The model under review builds one solid part; all positions refer to its coordinate system, in mm. A direction names the side the tool comes from. Give positions to 0.01 mm unless a question says otherwise; leave off trailing zeros. Loops run counter-clockwise (first coordinate to the right, second up) from the corner with the lowest first, then second, coordinate; pieces in that order, holes last. Notation, with made-up numbers: (36.25, -0.75) - (40.25, -0.75) arc R14 cw to (40.25, 8.25) - close; hole circle Ø1 at (-36.75, -38). An arc over 180 degrees is marked (long way). Return JSON: item names as keys, results as strings. Group by question number.
Autodesk Inventor part; units mm, degrees
ref_plane "YZ Plane" through (0, 0, 0) normal (1, 0, 0) x (0, 1, 0)
ref_plane "XZ Plane" through (0, 0, 0) normal (0, 1, 0) x (-1, 0, 0)
ref_plane "XY Plane" through (0, 0, 0) normal (0, 0, 1) x (1, 0, 0)
sketch "Sketch1" plane through (0, 0, 0) normal (0, 0, 1) x (1, 0, 0)
  circle A0 centre (0, 0) radius 10
  arc A1 (13.1244, -10) -> (-13.1244, -10) centre (0, 0) ccw
  line L0 (13.1244, -10) -> (25, -10)
  line L1 (25, -10) -> (0, -10)
  line L2 (-13.1244, -10) -> (-25, -10)
  line L3 (0, 0) -> (0, -17.5)
  line L4 (0, -17.5) -> (-25, -17.5)
  line L5 (-25, -17.5) -> (-25, -10)
  line L6 (25, -10) -> (25, -17.5)
  line L7 (25, -17.5) -> (0, -17.5)
  line L8 (0, 0) -> (-12.5, 0)
  circle A2 centre (-12.5, 0) radius 1.25
  line L9 (0, 0) -> (0, 12.5)
  circle A3 centre (0, 12.5) radius 1.25
  circle A4 centre (12.5, 0) radius 1.25
  circle A5 centre (0, -12.5) radius 1.25
  circle A6 centre (12.5, 0) radius 3.25
  circle A7 centre (-12.5, 0) radius 3.25
  line L10 (0, 0) -> (2.11, 2.11)
  line L11 (0, 0) -> (2.984, 0) construction
  circle A8 centre (0, 12.5) radius 3.25
  circle A9 centre (0, -12.5) radius 3.25
  dimension "d0" = 20
  dimension "d1" = 33
  dimension "d2" = 25
  dimension "d3" = 25
  dimension "d4" = 17.5
  dimension "d5" = 25
  dimension "d6" = 12.5
  dimension "d7" = 2.5
  dimension "d8" = 12.5
  dimension "d9" = 2.5
  dimension "d15" = 6.5
  dimension "d16" = 45
  dimension "d17" = 6.5
  dimension "d18" = 6.5
extrude "Extrusion1" add sketch "Sketch1" along normal blind 6 contours A0 A6 | A0 A8 A7 A9 L3 L4 L5 L2 A1 L1 A6 | A0 A8 | A9 L1 A0 | L3 A5 A9 A0 | L1 A9 L3 A5 | L1 L0 L6 L7 L3 A9 | A5 L3 | L3 A5 | A0 A7 picked at (10.6028, 1.4923)
fillet "Fillet1" radius 5 2 edges at (13.1244, -10, 3) (-13.1244, -10, 3)
sketch "Sketch2" plane through (0, 0, 0) normal (0, 0, -1) x (-1, 0, 0)
  circle A0 centre (0, 12.5) radius 1.25
  line L0 (0, 0) -> (-3.0567, 0)
  circle A1 centre (0, -12.5) radius 1.25
extrude "Extrusion2" cut sketch "Sketch2" against normal blind 10 contours A1
sketch "Sketch3" plane through (0, 0, 0) normal (0, 0, -1) x (-1, 0, 0)
  circle A0 centre (-12.5, 0) radius 1.25
  circle A1 centre (0, -12.5) radius 1.25
  circle A2 centre (0, 0) radius 10
  circle A3 centre (-12.5, 0) radius 1.25
  circle A4 centre (0, 12.5) radius 1.25
  circle A5 centre (12.5, 0) radius 1.25
  line L0 (25, -17.5) -> (-25, -17.5)
  line L1 (25, -10) -> (25, -17.5)
  line L2 (20.9105, -10) -> (25, -10)
  arc A6 (16.0476, -3.8372) -> (20.9105, -10) centre (20.9105, -5) ccw
  arc A7 (16.0476, -3.8372) -> (-16.0476, -3.8372) centre (0, 0) ccw
  arc A8 (-20.9105, -10) -> (-16.0476, -3.8372) centre (-20.9105, -5) ccw
  line L3 (-25, -10) -> (-20.9105, -10)
  line L4 (-25, -17.5) -> (-25, -10)
  circle A9 centre (-12.5, 0) radius 3.25
  circle A10 centre (0, 12.5) radius 3.25
  circle A11 centre (12.5, 0) radius 1.25
  circle A12 centre (12.5, 0) radius 3.25
  circle A13 centre (0, -12.5) radius 3.25
  dimension "d19" = 6.5
  dimension "d20" = 6.5
  dimension "d21" = 6.5
  dimension "d22" = 6.5
extrude "Extrusion3" cut sketch "Sketch3" against normal blind 3 contours A2 A12 | A2 A12 | A10 A2 | A2 A10 | A13 A2 | A2 A13 | A9 A2 | A2 A9
sketch "Sketch4" plane through (0, 0, 0) normal (0, 0, -1) x (-1, 0, 0)
  arc A0 (16.0476, -3.8372) -> (-16.0476, -3.8372) centre (0, 0) ccw
  line L0 (-25, -10) -> (-20.9105, -10)
  line L1 (-16.0476, 3.8372) -> (-20.9105, -10)
  line L2 (15.5959, 5.3868) -> (20.9105, -10)
  arc A1 (16.0476, -3.8372) -> (20.9105, -10) centre (20.9105, -5) ccw
  arc A2 (-20.9105, -10) -> (-16.0476, -3.8372) centre (-20.9105, -5) ccw
extrude "Extrusion4" add sketch "Sketch4" against normal up to surface (6 mm away)
sketch "Sketch5" plane through (-25, -17.5, 0) normal (0, -1, 0) x (1, 0, 0)
  line L0 (0, 6) -> (50, 6)
  line L1 (0, 0) -> (50, 0)
  circle A0 centre (40.75, 3) radius 1.25
  circle A1 centre (9.25, 3) radius 1.25
  point P0 (25, 0)
  dimension "d27" = 2.5
extrude "Extrusion5" cut sketch "Sketch5" against normal blind 14
sketch "Sketch6" plane through (-25, -17.5, 0) normal (0, -1, 0) x (1, 0, 0)
  circle A0 centre (9.25, 3) radius 1.25
  circle A1 centre (40.75, 3) radius 1.25
  point P0 (25, 0)
  dimension "d30" = 31.5
sketch "Sketch8" plane through (-25, -10, 6) normal (0, 1, 0) x (1, 0, 0)
  line L0 (9.4041, 6) -> (41.0476, 6)
  line L1 (4.0895, 6) -> (4.0895, 0)
  line L2 (9.4041, 6) -> (4.0895, 6)
  line L3 (4.0895, 6) -> (4.0895, 0)
  line L4 (4.0895, 0) -> (9.4041, 0)
  line L5 (9.4041, 0) -> (9.4041, 6)
  line L6 (45.8371, 0) -> (50, 0)
  line L7 (50, 0) -> (50, 6)
  line L8 (50, 6) -> (45.8371, 6)
  line L9 (45.8371, 6) -> (45.8371, 0)
  line L10 (0, 0) -> (4.0895, 0)
  line L11 (4.0895, 0) -> (4.0895, 6)
  line L12 (4.0895, 6) -> (0, 6)
  line L13 (0, 6) -> (0, 0)
  point P0 (25, 6)
extrude "Extrusion7" cut sketch "Sketch8" against normal blind 14 contours L1 L10 L13 L12 | L9 L8 L7 L6
sketch "Sketch9" plane through (0, 0, 0) normal (0, 0, -1) x (-1, 0, 0)
  arc A0 (-1.8494, 9.8275) -> (-9.8275, 1.8494) centre (0, 0) ccw
  arc A1 (-9.8275, 1.8494) -> (-9.8275, -1.8494) centre (0, 0) ccw
  arc A2 (-9.8275, -1.8494) -> (-1.8494, -9.8275) centre (0, 0) ccw
  arc A3 (-1.8494, -9.8275) -> (1.8494, -9.8275) centre (0, 0) ccw
  arc A4 (1.8494, -9.8275) -> (9.8275, -1.8494) centre (0, 0) ccw
  arc A5 (9.8275, -1.8494) -> (9.8275, 1.8494) centre (0, 0) ccw
  arc A6 (9.8275, 1.8494) -> (1.8494, 9.8275) centre (0, 0) ccw
  arc A7 (1.8494, 9.8275) -> (-1.8494, 9.8275) centre (0, 0) ccw
  circle A8 centre (0, 0) radius 8
  dimension "d37" = 16
extrude "Extrusion8" add sketch "Sketch9" against normal blind 4
sketch "Sketch11" plane through (0, 0, 0) normal (0, 0, -1) x (-1, 0, 0)
  arc A0 (-9.8275, 1.8494) -> (-9.8275, -1.8494) centre (-12.5, 0) ccw
  circle A1 centre (-12.5, 0) radius 3.25
  arc A2 (1.8494, 9.8275) -> (-1.8494, 9.8275) centre (0, 12.5) ccw
  arc A3 (9.8275, -1.8494) -> (9.8275, 1.8494) centre (0, 0) ccw
  arc A4 (9.8275, -1.8494) -> (9.8275, 1.8494) centre (12.5, 0) ccw
  circle A5 centre (12.5, 0) radius 1.25
  arc A6 (-1.8494, -9.8275) -> (1.8494, -9.8275) centre (0, 0) ccw
  arc A7 (-1.8494, -9.8275) -> (1.8494, -9.8275) centre (0, -12.5) ccw
  circle A8 centre (0, -12.5) radius 1.25
  circle A9 centre (0, 12.5) radius 3.25
  circle A10 centre (12.5, 0) radius 3.25
  circle A11 centre (0, -12.5) radius 3.25
extrude "Extrusion9" cut sketch "Sketch11" against normal up to surface (3 mm away)
sketch "Sketch12" plane through (0, 0, 0) normal (0, 0, -1) x (-1, 0, 0)
  line L0 (-20.8371, -10) -> (-20.8371, -17.5)
  arc A0 (-12.135, 11.18) -> (-20.8371, -10) centre (5.9768, -8.6392) ccw
  line L1 (-12.135, 11.18) -> (-20.8458, -9.8158)
  line L2 (0, 0) -> (0, 1.5642)
  arc A1 (20.8371, -10) -> (12.135, 11.18) centre (-5.9768, -8.6392) ccw
  line L3 (12.135, 11.18) -> (20.8458, -9.8158)
extrude "Extrusion10" add sketch "Sketch12" against normal up to surface (6 mm away)
properties part number "ROTATION1"
Item 1: Mouldability with a two-part tool opening along X and no side actions: class faces 5 (the face through (18.76, 1.8, 2.96)), 6 (the face through (-17, -11, 3)), 7 (the face through (-20.91, -14, 3)) as +X half, -X half, draft (parallel to the pull), parting line (faces both ways), or undercut.
Item 2: Take a section at A-A (y = -12.5). State the section outline as (x, z) points.
Item 3: Take a section at D-D (z = 0.7). State how many separate pieces and enclosed holes the cut face has, then the cut area to 3 significant figures.
Item 4: Take a section at C-C (y = 13). State the section outline as (x, z) points.
Item 5: Take a section at B-B (x = 0). State the section outline as (y, z) points.
Item 6: Tool access review of faces 1 (the face through (0, 8.2, 4)), 2 (the face through (-0.16, 11.26, 4.48)), 3 (the face through (-16, -3.5, 3)), 4 (the face through (0, 11, 3)): name each direction out of +Z, -Z, +X, -X, +Y, -Y from which nothing blocks a thin tool from reaching the whole face with its end or side.
Item 7: For P1, Ø2, axis at y = 3.5, z = 3, coming from the +X side; P2, Ø1.5, axis at x = -15.75, z = 3, coming from the +Y side; P3, Ø2, axis at x = -0.5, y = 12.5, coming from the -Z side, all flat-tipped, find the tip position at first contact; note any pin that passes through.
Item 8: For L1, parallel to Y at x = 0, z = 1.75; L2, parallel to X at y = -4.5, z = 2.5; L3, parallel to Y at x = -4, z = 0.3, list the stretches that pass through material, from the lowest coordinate up. Write a range as from..to.
Check sheet entries:
{
 "1": {"face 5": "+X half", "face 6": "undercut", "face 7": "-X half"},
 "2": {"outline": "(-20.91, 0) - (-3.25, 0) - (-3.25, 3) - (-1.25, 3) - (-1.25, 6) - (-20.91, 6) - close; (1.25, 3) - (3.25, 3) - (3.25, 0) - (20.84, 0) - (20.84, 6) - (1.25, 6) - close; hole circle Ø2.5 at (-15.75, 3); hole circle Ø2.5 at (15.75, 3)"},
 "3": {"separate pieces": "1", "enclosed holes": "5", "area": "846 mm^2"},
 "4": {"outline": "(-10.16, 0) - (-3.21, 0) - (-3.21, 3) - (-1.15, 3) - (-1.15, 6) - (-10.16, 6) - close; (1.15, 3) - (3.21, 3) - (3.21, 0) - (10.16, 0) - (10.16, 6) - (1.15, 6) - close"},
 "5": {"outline": "(-17.5, 0) - (-15.75, 0) - (-15.75, 3) - (-13.75, 3) - (-13.75, 6) - (-17.5, 6) - close; (-11.25, 3) - (-9.25, 3) - (-9.25, 0) - (-8, 0) - (-8, 4) - (-10, 4) - (-10, 6) - (-11.25, 6) - close; (8, 0) - (9.25, 0) - (9.25, 3) - (11.25, 3) - (11.25, 6) - (10, 6) - (10, 4) - (8, 4) - close; (13.75, 3) - (15.75, 3) - (15.75, 0) - (16.5, 0) - (16.5, 6) - (13.75, 6) - close"},
 "6": {"face 1": "+Z", "face 2": "+Z, -Z", "face 3": "-Y", "face 4": "-Z"},
 "7": {"P1": "stops at x = 18.45", "P2": "stops at y = 8.12", "P3": "stops at z = 3"},
 "8": {"L1": "y = -17.5..-15.75, -9.25..-8, 8..9.25, 15.75..16.5", "L2": "x = -20.55..-16.9, -14.6..-6.61, 6.61..14.6, 16.9..20.55", "L3": "y = -17.5..-6.93, 6.93..16.01"}
}
